CAD build for the part. Positions are in the model's coordinates, mm. A direction names the side the tool comes from. Coordinates: 2 decimals unless noted, no trailing zeros. Loops run counter-clockwise (first coordinate to the right, second up) from the corner with the lowest first, then second, coordinate; pieces in that order, holes last. Notation, with made-up numbers: (65, 85) -> (71, 85) arc R20 cw to (71, 123) -> close; hole circle Ø7 at (57, 86.25). An arc over 180 degrees is marked (long way). Answer as CSV lines item,"result". Start each with the question number.
```python
from build123d import *

# Parameters (mm, degrees)
F1_DEPTH = 40
F3_DEPTH = 360
F4_R     = 5


with BuildPart() as f1:
    # F0 (on Top) → F1 (new body)
    with BuildSketch(Plane.XY):
        with BuildLine():
            Line((179.756029, 214.536132), (-180.243971, 214.536132))
            ThreePointArc((-180.243971, 214.536132), (-194.386107, 208.678267), (-200.243971, 194.536132))
            Line((-200.243971, 194.536132), (-200.243971, -165.463868))
            ThreePointArc((-200.243971, -165.463868), (-194.386107, -179.606004), (-180.243971, -185.463868))
            Line((-180.243971, -185.463868), (179.756029, -185.463868))
            ThreePointArc((179.756029, -185.463868), (193.898164, -179.606004), (199.756029, -165.463868))
            Line((199.756029, -165.463868), (199.756029, 194.536132))
            ThreePointArc((199.756029, 194.536132), (193.898164, 208.678267), (179.756029, 214.536132))
        make_face()
    extrude(amount=F1_DEPTH)

    # F2 (on face) → F3 (join)
    with BuildSketch(Plane(origin=(0, 0, 0), x_dir=(1, 0, 0), z_dir=(0, 0, -1))):
        with BuildLine():
            Line((-125.243971, 145.463868), (-155.243971, 145.463868))
            ThreePointArc((-155.243971, 145.463868), (-158.779505, 143.999402), (-160.243971, 140.463868))
            Line((-160.243971, 140.463868), (-160.243971, 110.463868))
            ThreePointArc((-160.243971, 110.463868), (-158.779505, 106.928334), (-155.243971, 105.463868))
            Line((-155.243971, 105.463868), (-125.243971, 105.463868))
            ThreePointArc((-125.243971, 105.463868), (-121.708437, 106.928334), (-120.243971, 110.463868))
            Line((-120.243971, 110.463868), (-120.243971, 140.463868))
            ThreePointArc((-120.243971, 140.463868), (-121.708437, 143.999402), (-125.243971, 145.463868))
        make_face()
        with BuildLine():
            Line((-125.243971, -134.536132), (-155.243971, -134.536132))
            ThreePointArc((-155.243971, -134.536132), (-158.779505, -136.000598), (-160.243971, -139.536132))
            Line((-160.243971, -139.536132), (-160.243971, -169.536132))
            ThreePointArc((-160.243971, -169.536132), (-158.779505, -173.071666), (-155.243971, -174.536132))
            Line((-155.243971, -174.536132), (-125.243971, -174.536132))
            ThreePointArc((-125.243971, -174.536132), (-121.708437, -173.071666), (-120.243971, -169.536132))
            Line((-120.243971, -169.536132), (-120.243971, -139.536132))
            ThreePointArc((-120.243971, -139.536132), (-121.708437, -136.000598), (-125.243971, -134.536132))
        make_face()
        with BuildLine():
            Line((154.756029, -134.536132), (124.756029, -134.536132))
            ThreePointArc((124.756029, -134.536132), (121.220495, -136.000598), (119.756029, -139.536132))
            Line((119.756029, -139.536132), (119.756029, -169.536132))
            ThreePointArc((119.756029, -169.536132), (121.220495, -173.071666), (124.756029, -174.536132))
            Line((124.756029, -174.536132), (154.756029, -174.536132))
            ThreePointArc((154.756029, -174.536132), (158.291563, -173.071666), (159.756029, -169.536132))
            Line((159.756029, -169.536132), (159.756029, -139.536132))
            ThreePointArc((159.756029, -139.536132), (158.291563, -136.000598), (154.756029, -134.536132))
        make_face()
        with BuildLine():
            Line((154.756029, 145.463868), (124.756029, 145.463868))
            ThreePointArc((124.756029, 145.463868), (121.220495, 143.999402), (119.756029, 140.463868))
            Line((119.756029, 140.463868), (119.756029, 110.463868))
            ThreePointArc((119.756029, 110.463868), (121.220495, 106.928334), (124.756029, 105.463868))
            Line((124.756029, 105.463868), (154.756029, 105.463868))
            ThreePointArc((154.756029, 105.463868), (158.291563, 106.928334), (159.756029, 110.463868))
            Line((159.756029, 110.463868), (159.756029, 140.463868))
            ThreePointArc((159.756029, 140.463868), (158.291563, 143.999402), (154.756029, 145.463868))
        make_face()
    extrude(amount=F3_DEPTH)

    # F4
    f4_edges = [f1.edges().sort_by_distance(p)[0] for p in [
        (199.756029, 14.536132, 40),
        (193.898164, 208.678267, 40),
        (-0.243971, 214.536132, 40),
        (-194.386107, 208.678267, 40),
        (-200.243971, 14.536132, 40),
        (-194.386107, -179.606004, 40),
        (-0.243971, -185.463868, 40),
        (193.898164, -179.606004, 40),
    ]]
    fillet(f4_edges, radius=F4_R)


solid = f1.part
```
Q1. Saw through at B-B (y = 121). List the corners of the cut face in (x, z).
Q2. Saw through at A-A (z = -151). Give the number of separate pieces and of enclosed holes in the cut face, and give its area (3 significant figures).
Q3. Saw through at C-C (x = -172.5). List the corners of the cut face in (y, z), and give its area (3 significant figures).
Q4. Probe probe 1 along X at (y, z) = (-127, -82.5); probe 2 along Y at (x, z) = (-144, -235.5); probe 3 along Z at (x, y) = (173, 173). List the from-to ranges inside material, lowest first. Write a range as from..to.
Q5. Two-plate mould, pull along X, no slides. Class faces 1 (the flat face through (140, 134.536, -177)), 2 (the flat face through (119.756, 154, -177)), 3 (the flat face through (-160.244, 154, -177)): pulls with the +X half, pulls with the -X half, needs draft (parallel to the pull), parting line crosses it, or undercut.
Q6. Pin check, flat tips, straight feed: pin 1 Ø9 at (y, z) = (159.5, -161.5) entering from +X; pin 2 Ø24 at (y, z) = (147.5, -136.5) entering from -X; pin 3 Ø10 at (x, z) = (139, -280) entering from +Y. Stop position of each tip, or through.
Q7. Which spindle directions (+Z, -Z, +X, -X, +Y, -Y) get a long thin tool onto all of the face, cutting with end or side? Do faces 4 (the flat face through (-140, 134.536, -177)), 5 (the flat face through (-140, -145.464, -177)), 6 (the flat face through (159.756, 155, -177)). Say none if no direction does.
Ans:
1,outline,"(-200.24, 0) -> (199.76, 0) -> (199.76, 35) arc R5 ccw to (194.76, 40) -> (-195.24, 40) arc R5 ccw to (-200.24, 35) -> close"
2,separate pieces,"4"
2,enclosed holes,"0"
2,area,"6,310 mm²"
3,outline,"(-185.46, 0) -> (214.54, 0) -> (214.54, 35) arc R5 ccw to (209.54, 40) -> (-180.46, 40) arc R5 ccw to (-185.46, 35) -> close"
3,area,"16,000 mm²"
4,probe 1,"x = -160.24..-120.24, 119.76..159.76"
4,probe 2,"y = -145.46..-105.46, 134.54..174.54"
4,probe 3,"z = 0..40"
5,face 1,"needs draft"
5,face 2,"undercut"
5,face 3,"pulls with the -X half"
6,pin 1,"stops at x = 159.76"
6,pin 2,"stops at x = -160.24"
6,pin 3,"stops at y = 174.54"
7,face 4,"-Z, +X, -X"
7,face 5,"-Z, +X, -X, -Y"
7,face 6,"-Z, +X, +Y, -Y"
